Model file for the job. Use its own axes, mm. A direction names the side the tool comes from. Coordinates: 2 decimals unless noted, no trailing zeros. Write each loop counter-clockwise with the first axis right and the second up, starting at its lowest first coordinate (ties: lowest second). Pieces come first, ordered by that corner, then holes.
Q1. Pin check, flat tips, straight feed: P1, Ø1.5, axis at x = 19, y = -7.5, coming from the +Z side; P2, Ø1.9, axis at x = -18.669, z = 82.169, coming from the -Y side; P3, Ø11, axis at x = -37, z = 53.5, coming from the -Y side; P4, Ø12, axis at y = -0.5, z = 23, coming from the -X side. Stop position of each tip, or through.
Q2. Band-saw the part on A-A, the plane x = 0. Write the cut outline in (y, z) (3 decimals), plus the area to 3 significant figures.
Q3. Which spindle directions (+Z, -Z, +X, -X, +Y, -Y) get a long thin tool onto all of the face, cutting with end or side? Do faces 4 (the cylindrical face through (19.76, 28.68, 5.58)), 5 (the cylindrical face through (27.84, -25.58, 79.18)), 6 (the cylindrical face through (-15.58, -32.39, 9.72)). Say none if no direction does.
Q4. Pull direction X, two halves, no side cores. Call faces 1 (the cylindrical face through (-19.82, 28.68, 5.64)), 2 (the cylindrical face through (-27.89, 5.68, 79.08)), 3 (the flat face through (-41, 27, 42)): released by +X, released by -X, zero draft, split by the parting line, or undercut.
Q5. Band-saw the part on B-B, the plane z = 55.5. State how many separate pieces and enclosed holes the cut face has, plus the area to 3 significant figures.
Q6. Drill centre lines: probe 1 along X at (y, z) = (-28, 43.5); probe 2 along Y at (x, z) = (0, -2); probe 3 along Y at (x, z) = (-24, 68.5). Where is each one in solid material? Low to high.
from build123d import *

# Parameters (mm, degrees)
BOSS_EXTRUDE1_DEPTH = 88.9
CUT_EXTRUDE5_DEPTH  = 73
CUT_EXTRUDE6_DEPTH  = 65.81
SKETCH8_W           = 52
SKETCH8_H           = 54.81
CUT_EXTRUDE7_DEPTH  = 15.875
SKETCH12_W          = 52
SKETCH12_H          = 54.81
CUT_EXTRUDE11_DEPTH = 63.5
SKETCH18_W          = 52
SKETCH18_H          = 54.81
CUT_EXTRUDE14_DEPTH = 81.026
BOSS_EXTRUDE2_DEPTH = 6.35
SKETCH20_R          = 2.5527
CUT_EXTRUDE15_DEPTH = 9.525
CUT_EXTRUDE16_DEPTH = 73
CUT_EXTRUDE17_DEPTH = 1.27
CUT_EXTRUDE18_DEPTH = 1.27
CUT_EXTRUDE19_DEPTH = 1.27
CUT_EXTRUDE20_DEPTH = 1.27


with BuildPart() as part:
    # Sketch1 → Boss-Extrude1 (new body)
    with BuildSketch(Plane.XY):
        Polygon((-41, 29.31), (41, 29.31), (41, 25.5), (31, 25.5), (31, -35.5), (-31, -35.5), (-31, 25.5), (-41, 25.5), align=None)
    extrude(amount=BOSS_EXTRUDE1_DEPTH)

    # Sketch6 → Cut-Extrude5 (cut, through all)
    with BuildSketch(Plane.ZY.offset(31)):
        with BuildLine():
            Line((14.351, 7.526), (74.549, 7.526))
            ThreePointArc((74.549, 7.526), (79.128930622, 5.628930622), (81.026, 1.049))
            Line((81.026, 1.049), (81.026, -21.049))
            ThreePointArc((81.026, -21.049), (79.128930622, -25.628930622), (74.549, -27.526))
            Line((74.549, -27.526), (14.351, -27.526))
            ThreePointArc((14.351, -27.526), (9.771069378, -25.628930622), (7.874, -21.049))
            Line((7.874, -21.049), (7.874, 1.049))
            ThreePointArc((7.874, 1.049), (9.771069378, 5.628930622), (14.351, 7.526))
        make_face()
    extrude(amount=-CUT_EXTRUDE5_DEPTH, mode=Mode.SUBTRACT)

    # Sketch7 → Cut-Extrude6 (cut, through all)
    with BuildSketch(Plane(origin=(0, -35.5, 0), x_dir=(0, 0, 1), z_dir=(0, -1, 0))):
        with BuildLine():
            Line((14.351, 17.526), (74.549, 17.526))
            ThreePointArc((74.549, 17.526), (79.128930622, 15.628930622), (81.026, 11.049))
            Line((81.026, 11.049), (81.026, -11.049))
            ThreePointArc((81.026, -11.049), (79.128930622, -15.628930622), (74.549, -17.526))
            Line((74.549, -17.526), (14.351, -17.526))
            ThreePointArc((14.351, -17.526), (9.771069378, -15.628930622), (7.874, -11.049))
            Line((7.874, -11.049), (7.874, 11.049))
            ThreePointArc((7.874, 11.049), (9.771069378, 15.628930622), (14.351, 17.526))
        make_face()
    extrude(amount=-CUT_EXTRUDE6_DEPTH, mode=Mode.SUBTRACT)

    # Sketch8 → Cut-Extrude7 (cut)
    with BuildSketch(Plane.XY.offset(88.9)):
        with Locations((0, -3.095)):
            Rectangle(SKETCH8_W, SKETCH8_H)
    extrude(amount=-CUT_EXTRUDE7_DEPTH, mode=Mode.SUBTRACT)

    # Sketch12 → Cut-Extrude11 (cut)
    with BuildSketch(Plane.XY.offset(88.9)):
        with Locations((0, -3.095)):
            Rectangle(SKETCH12_W, SKETCH12_H)
    extrude(amount=-CUT_EXTRUDE11_DEPTH, mode=Mode.SUBTRACT)

    # Sketch18 → Cut-Extrude14 (cut)
    with BuildSketch(Plane.XY.offset(88.9)):
        with Locations((0, -3.095)):
            Rectangle(SKETCH18_W, SKETCH18_H)
    extrude(amount=-CUT_EXTRUDE14_DEPTH, mode=Mode.SUBTRACT)

    # Sketch19 → Boss-Extrude2 (add)
    with BuildSketch(Plane(origin=(0, 0, 0), x_dir=(-1, 0, 0), z_dir=(0, 0, -1))):
        Polygon((31, 25.5), (41, 25.5), (41, 29.31), (-41, 29.31), (-41, 25.5), (-31, 25.5), (-31, -35.5), (31, -35.5), align=None)
    extrude(amount=BOSS_EXTRUDE2_DEPTH)

    # Sketch20 → Cut-Extrude15 (cut)
    with BuildSketch(Plane(origin=(0, 0, -6.35), x_dir=(-1, 0, 0), z_dir=(0, 0, -1))):
        with Locations((0, -4.844639258)):
            Circle(SKETCH20_R)
    extrude(amount=-CUT_EXTRUDE15_DEPTH, mode=Mode.SUBTRACT)

    # Sketch21 → Cut-Extrude16 (cut, through all)
    with BuildSketch(Plane(origin=(31, 0, 0), x_dir=(0, 0, -1), z_dir=(1, 0, 0))):
        with BuildLine():
            Line((6.35, -4), (6.35, -6))
            ThreePointArc((6.35, -6), (5.35, -5), (6.35, -4))
        make_face()
    extrude(amount=-CUT_EXTRUDE16_DEPTH, mode=Mode.SUBTRACT)

    # Sketch22 → Cut-Extrude17 (cut)
    with BuildSketch(Plane(origin=(0, -35.5, 0), x_dir=(-1, 0, 0), z_dir=(0, -1, 0))):
        with BuildLine():
            Line((-17.164974651, -6.223), (17.164974651, -6.223))
            ThreePointArc((17.164974651, -6.223), (19.791532015, -5.608467985), (19.177, -8.235025349))
            Line((19.177, -8.235025349), (19.177, -80.664974651))
            ThreePointArc((19.177, -80.664974651), (19.791532015, -83.291532015), (17.164974651, -82.677))
            Line((17.164974651, -82.677), (-17.164974651, -82.677))
            ThreePointArc((-17.164974651, -82.677), (-19.791532015, -83.291532015), (-19.177, -80.664974651))
            Line((-19.177, -80.664974651), (-19.177, -8.235025349))
            ThreePointArc((-19.177, -8.235025349), (-19.791532015, -5.608467985), (-17.164974651, -6.223))
        make_face()
    extrude(amount=-CUT_EXTRUDE17_DEPTH, mode=Mode.SUBTRACT)

    # Sketch23 → Cut-Extrude18 (cut)
    with BuildSketch(Plane(origin=(-31, 0, 0), x_dir=(0, 1, 0), z_dir=(-1, 0, 0))):
        with BuildLine():
            Line((-27.164974651, -6.223), (7.164974651, -6.223))
            ThreePointArc((7.164974651, -6.223), (9.791532015, -5.608467985), (9.177, -8.235025349))
            Line((9.177, -8.235025349), (9.177, -80.664974651))
            ThreePointArc((9.177, -80.664974651), (9.791532015, -83.291532015), (7.164974651, -82.677))
            Line((7.164974651, -82.677), (-27.164974651, -82.677))
            ThreePointArc((-27.164974651, -82.677), (-29.791532015, -83.291532015), (-29.177, -80.664974651))
            Line((-29.177, -80.664974651), (-29.177, -8.235025349))
            ThreePointArc((-29.177, -8.235025349), (-29.791532015, -5.608467985), (-27.164974651, -6.223))
        make_face()
    extrude(amount=-CUT_EXTRUDE18_DEPTH, mode=Mode.SUBTRACT)

    # Sketch24 → Cut-Extrude19 (cut)
    with BuildSketch(Plane(origin=(31, 0, 0), x_dir=(0, -1, 0), z_dir=(1, 0, 0))):
        with BuildLine():
            Line((-7.164974651, -6.223), (27.164974651, -6.223))
            ThreePointArc((27.164974651, -6.223), (29.791532015, -5.608467985), (29.177, -8.235025349))
            Line((29.177, -8.235025349), (29.177, -80.664974651))
            ThreePointArc((29.177, -80.664974651), (29.791532015, -83.291532015), (27.164974651, -82.677))
            Line((27.164974651, -82.677), (-7.164974651, -82.677))
            ThreePointArc((-7.164974651, -82.677), (-9.791532015, -83.291532015), (-9.177, -80.664974651))
            Line((-9.177, -80.664974651), (-9.177, -8.235025349))
            ThreePointArc((-9.177, -8.235025349), (-9.791532015, -5.608467985), (-7.164974651, -6.223))
        make_face()
    extrude(amount=-CUT_EXTRUDE19_DEPTH, mode=Mode.SUBTRACT)

    # Sketch25 → Cut-Extrude20 (cut)
    with BuildSketch(Plane(origin=(0, 29.31, 0), x_dir=(1, 0, 0), z_dir=(0, 1, 0))):
        with BuildLine():
            Line((-17.164974651, -6.223), (17.164974651, -6.223))
            ThreePointArc((17.164974651, -6.223), (19.791532015, -5.608467985), (19.177, -8.235025349))
            Line((19.177, -8.235025349), (19.177, -80.664974651))
            ThreePointArc((19.177, -80.664974651), (19.791532015, -83.291532015), (17.164974651, -82.677))
            Line((17.164974651, -82.677), (-17.164974651, -82.677))
            ThreePointArc((-17.164974651, -82.677), (-19.791532015, -83.291532015), (-19.177, -80.664974651))
            Line((-19.177, -80.664974651), (-19.177, -8.235025349))
            ThreePointArc((-19.177, -8.235025349), (-19.791532015, -5.608467985), (-17.164974651, -6.223))
        make_face()
    extrude(amount=-CUT_EXTRUDE20_DEPTH, mode=Mode.SUBTRACT)


solid = part.part
Answer sheet:
1. P1: stops at z = 7.87
1. P2: stops at y = -34.23
1. P3: stops at y = 25.5
1. P4: passes through
2. outline: (-35.5, -6.35) - (-7.397, -6.35) - (-7.397, 3.175) - (-2.292, 3.175) - (-2.292, -6.35) - (29.31, -6.35) - (29.31, 6.223) - (28.04, 6.223) - (28.04, 7.874) - (-34.23, 7.874) - (-34.23, 6.223) - (-35.5, 6.223) - close; (-35.5, 82.677) - (-34.23, 82.677) - (-34.23, 81.026) - (-30.5, 81.026) - (-30.5, 88.9) - (-35.5, 88.9) - close; (24.31, 81.026) - (28.04, 81.026) - (28.04, 82.677) - (29.31, 82.677) - (29.31, 88.9) - (24.31, 88.9) - close
2. area: 944 mm2
3. face 4: +Y
3. face 5: +X, -X
3. face 6: +Y, -Y
4. face 1: undercut
4. face 2: zero draft
4. face 3: released by -X
5. separate pieces: 4
5. enclosed holes: 0
5. area: 526 mm2
6. probe 1: x = -29.73 to -26, 26 to 29.73
6. probe 2: y = -35.5 to -7.4, -2.29 to 29.31
6. probe 3: y = -35.5 to -30.5, 24.31 to 29.31
